```python
from build123d import *

# Parameters (mm, degrees)
F1_DEPTH = 33
F2_SIZE  = 5
F3_SIZE  = 5


with BuildPart() as f1:
    # F0 (on Front) → F1 (new body)
    with BuildSketch(Plane.XZ):
        Polygon((0, 81.5), (0, 0), (13, 0), (13, 54), (189.5, 54), (189.5, 0), (202.5, 0), (202.5, 81.5), (135, 81.5), (135, 94), (120, 94), (120, 81.5), align=None)
    extrude(amount=F1_DEPTH)

    # F2
    f2_edges = [f1.edges().sort_by_distance(p)[0] for p in [
        (6.5, -33, 0),
    ]]
    chamfer(f2_edges, length=F2_SIZE)

    # F3
    f3_edges = [f1.edges().sort_by_distance(p)[0] for p in [
        (196, -33, 0),
    ]]
    chamfer(f3_edges, length=F3_SIZE)


solid = f1.part
```
For this review, take the finished solid that the model builds, in its own axes (mm). A direction names the side the tool comes from. Coordinates: 2 decimals unless noted, no trailing zeros. Loops run counter-clockwise (first coordinate to the right, second up) from the corner with the lowest first, then second, coordinate; pieces in that order, holes last. Notation, with made-up numbers: (65.5, 30) -> (114.5, 30) arc R17 cw to (114.5, 62) -> close; hole circle Ø9 at (-12, 68). An arc over 180 degrees is marked (long way). Return JSON: item names as keys, results as strings. Group by question number.
(1) Consider section D-D, the plane y = -30. Give the boundary of the cut face in (x, z), plus the area to 3 significant figures.
(2) Consider section A-A, the plane z = 47.5. Give the boundary of the cut face in (x, y).
(3) To check wall thickness, follow L1, parallel to X at y = -3, z = 39.5; L2, parallel to Z at x = 128.5, y = -26; L3, parallel to Z at x = 56.5, y = -13.5. State the ranges of each line that lie inside material, in increasing order.
(4) Consider section B-B, the plane y = -15.5. Give the boundary of the cut face in (x, z).
(5) Consider section C-C, the plane x = 123.5. Give the boundary of the cut face in (y, z).
(6) Tool access review of faces 4 (the flat face through (169, -16, 81.5)), 5 (the flat face through (100, -16, 54)), 6 (the flat face through (0, -16, 41)), 7 (the flat face through (61, -16, 81.5)): name each direction out of +Z, -Z, +X, -X, +Y, -Y from which nothing blocks a thin tool from reaching the whole face with its end or side.
(7) Mouldability with a two-part tool opening along X and no side actions: class faces 1 (the flat face through (135, -16, 88)), 2 (the flat face through (128, -16, 94)), 3 (the flat face through (13, -16, 27)) as pulls with the +X half, pulls with the -X half, needs draft (parallel to the pull), parting line crosses it, or undercut.
(8) For pin 1 Ø10 at (x, y) = (164, -22.5) entering from +Z; pin 2 Ø6 at (y, z) = (-21, 86) entering from -X; pin 3 Ø8 at (x, y) = (99, -12) entering from -Z, all flat-tipped, find the tip position at first contact; note any pin that passes through.
Results below:
{
 "1": {"outline": "(0, 2) -> (13, 2) -> (13, 54) -> (189.5, 54) -> (189.5, 2) -> (202.5, 2) -> (202.5, 81.5) -> (135, 81.5) -> (135, 94) -> (120, 94) -> (120, 81.5) -> (0, 81.5) -> close", "area": "7,110 mm2"},
 "2": {"outline": "(0, -33) -> (13, -33) -> (13, 0) -> (0, 0) -> close; (189.5, -33) -> (202.5, -33) -> (202.5, 0) -> (189.5, 0) -> close"},
 "3": {"L1": "x = 0 to 13, 189.5 to 202.5", "L2": "z = 54 to 94", "L3": "z = 54 to 81.5"},
 "4": {"outline": "(0, 0) -> (13, 0) -> (13, 54) -> (189.5, 54) -> (189.5, 0) -> (202.5, 0) -> (202.5, 81.5) -> (135, 81.5) -> (135, 94) -> (120, 94) -> (120, 81.5) -> (0, 81.5) -> close"},
 "5": {"outline": "(-33, 54) -> (0, 54) -> (0, 94) -> (-33, 94) -> close"},
 "6": {"face 4": "+Z, +X, +Y, -Y", "face 5": "-Z, +Y, -Y", "face 6": "+Z, -Z, -X, +Y, -Y", "face 7": "+Z, -X, +Y, -Y"},
 "7": {"face 1": "pulls with the +X half", "face 2": "needs draft", "face 3": "undercut"},
 "8": {"pin 1": "stops at z = 81.5", "pin 2": "stops at x = 120", "pin 3": "stops at z = 54"}
}
